Read the model definition and answer for the solid it produces. Units are mm, in the model's axes. A direction names the side the tool comes from. Coordinates: 2 decimals unless noted, no trailing zeros. Loops run counter-clockwise (first coordinate to the right, second up) from the corner with the lowest first, then second, coordinate; pieces in that order, holes last. Notation, with made-up numbers: (30.25, 22) -> (88.25, 22) arc R10 ccw to (88.25, 29) -> close; hole circle Ø10 at (71, 35). An arc over 180 degrees is marked (long way). Answer as CSV lines item,"result".
```python
from build123d import *

# Parameters (mm, degrees)
F0_W     = 10
F0_H     = 10.306037739
F1_DEPTH = 3
F3_DEPTH = 3
F4_W     = 10
F4_H     = 5.1530188695
F5_DEPTH = 3
F6_W     = 5
F6_H     = 5.1530188695
F7_DEPTH = 3
F8_R     = 1
F8_W     = 0.8780423959
F8_H     = 0.9329200257
F8_W_2   = 0.8780424541
F8_H_2   = 0.9603588842
F9_DEPTH = 3
F10_R    = 1


with BuildPart() as f1:
    # F0 (on Top) → F1 (new body)
    with BuildSketch(Plane.XY):
        Rectangle(F0_W, F0_H)
    extrude(amount=F1_DEPTH)

    # F2 (on face) → F3 (join)
    with BuildSketch(Plane.XY.offset(3)):
        Polygon((-5, 5.1530188695), (-5, 0), (0, 0), (0, -5.1530188695), (5, -5.1530188695), (5, 5.1530188695), (-2.5035347862, 5.1530188695), align=None)
    extrude(amount=F3_DEPTH)

    # F4 (on face) → F5 (join)
    with BuildSketch(Plane.XY.offset(6)):
        with Locations((0, 2.5765094348)):
            Rectangle(F4_W, F4_H)
    extrude(amount=F5_DEPTH)

    # F6 (on face) → F7 (join)
    with BuildSketch(Plane.XY.offset(9)):
        with Locations((-2.5, 2.5765094348)):
            Rectangle(F6_W, F6_H)
    extrude(amount=F7_DEPTH)

    # F8 (on face) → F9 (cut)
    with BuildSketch(Plane(origin=(0, 5.1530188695, 0), x_dir=(-1, 0, 0), z_dir=(0, 1, 0))):
        with Locations((-2.5, 7.5359190814)):
            Circle(F8_R)
        with Locations((-2.5, 4.5)):
            Circle(F8_R)
        with Locations((-2.5, 1.4719393803)):
            Circle(F8_R)
        with Locations((-0.7341963501, 2.9536358779)):
            Rectangle(F8_W, F8_H)
        with Locations((-0.734196321, 6.0405035038)):
            Rectangle(F8_W_2, F8_H_2)
        Polygon((1.1865213746, 11.4322323352), (0, 0.7859683246), (2.8032438053, 0.729703495), (4.2047919706, 2.322542714), (1.7662906772, 2.322542714), (4.2047919706, 5.0938641652), (1.7662906772, 5.0938641652), (4.2047919706, 7.3987250216), (1.7662906772, 7.3987250216), (4.2047919706, 9.5562967831), (1.7662906772, 9.5562967831), (4.2047919706, 11.4322323352), align=None)
    extrude(amount=-F9_DEPTH, mode=Mode.SUBTRACT)

    # F10
    f10_edges = [f1.edges().sort_by_distance(p)[0] for p in [
        (-5, 2.576509, 12),
        (5, 2.576509, 9),
        (0, -2.576509, 6),
        (-5, -2.576509, 3),
    ]]
    fillet(f10_edges, radius=F10_R)


solid = f1.part
```
Q1. A cutting plane is placed at C-C, the plane z = 4. Write down the section's boundary in (x, y), and give its area (3 significant figures).
Results:
outline,"(-5, 0) -> (0, 0) -> (0, -5.15) -> (5, -5.15) -> (5, 5.15) -> (3.37, 5.15) -> (3.37, 2.15) -> (1.63, 2.15) -> (1.63, 5.15) -> (-0.36, 5.15) -> (-0.36, 2.15) -> (-3.24, 2.15) -> (-3.24, 5.15) -> (-5, 5.15) -> close"
area,"63.4 mm²"
Q2. Find the intervals of material crossed by probe 1 along Z at (x, y) = (2.5, 3.4); probe 2 along Z at (x, y) = (3.25, 2.5); probe 3 along X at (y, z) = (2.5, 1.25), in increasing order. Write a range as [from, to].
Results:
probe 1,"z = [0, 0.47], [2.47, 3.5], [5.5, 6.54], [8.54, 9]"
probe 2,"z = [0, 0.81], [2.13, 3.84], [5.16, 6.87], [8.2, 9]"
probe 3,"x = [-5, -3.26], [-0.05, 1.52], [3.48, 5]"
Q3. A cutting plane is placed at A-A, the plane x = 2.5. Write down the section's boundary in (y, z), and give its area (3 significant figures).
Results:
outline,"(-5.15, 0) -> (5.15, 0) -> (5.15, 0.47) -> (2.15, 0.47) -> (2.15, 2.47) -> (5.15, 2.47) -> (5.15, 3.5) -> (2.15, 3.5) -> (2.15, 5.5) -> (5.15, 5.5) -> (5.15, 6.54) -> (2.15, 6.54) -> (2.15, 8.54) -> (5.15, 8.54) -> (5.15, 9) -> (0, 9) -> (0, 6) -> (-5.15, 6) -> close"
area,"59.3 mm²"
Q4. A cutting plane is placed at B-B, the plane y = 4. Give the number of separate pieces and of enclosed holes in the cut face, and give its area (3 significant figures).
Results:
separate pieces,"1"
enclosed holes,"6"
area,"67.1 mm²"
Q5. Given pin 1 Ø4 at (x, y) = (2.5, -3.5) entering from +Z; pin 2 Ø2 at (y, z) = (-3.5, 4.5) entering from -X; pin 3 Ø0.7 at (x, y) = (0.5, 4) entering from +Z, each flat-ended and moving along its own axis, determine where each tip first touches the part or whether it passes through.
Results:
pin 1,"stops at z = 6"
pin 2,"stops at x = 0"
pin 3,"stops at z = 9"
Q6. For a pull along Z with two mould halves and no side action, classify faces 1 (the face through (-2, 2.153, 6)), 2 (the face through (0, 5.153, 6)), 3 (the face through (0.285, -2.613, 5.699)) as pulls with the +Z half, pulls with the -Z half, needs draft (parallel to the pull), parting line crosses it, or undercut.
Results:
face 1,"undercut"
face 2,"needs draft"
face 3,"pulls with the +Z half"
Q7. For faces 4 (the face through (4.699, 2.613, 8.715)), 5 (the face through (-3, 4, 11.432)), determine the directions among +Z, -Z, +X, -X, +Y, -Y from which every point of the face is accessible in a straight line to the end or side of a thin tool.
Results:
face 4,"+Z, +X, +Y, -Y"
face 5,"+Y"
Q8. A cutting plane is placed at D-D, the plane y = 1. Write down the section's boundary in (x, z), and give its area (3 significant figures).
Results:
outline,"(-5, 0) -> (5, 0) -> (5, 8) arc R1 ccw to (4, 9) -> (0, 9) -> (0, 12) -> (-4, 12) arc R1 ccw to (-5, 11) -> close"
area,"105 mm²"
